Source: three-view drawing plus pictorial views. Frame: mm from the lowest corner of the part. A direction names the side the tool comes from. Give positions to 0.01 mm unless a question says otherwise; leave off trailing zeros. Loops run counter-clockwise (first coordinate to the right, second up) from the corner with the lowest first, then second, coordinate; pieces in that order, holes last. Notation, with made-up numbers: (-25.75, -28) -> (-13.75, -28) arc R26 cw to (-13.75, 5) -> close; hole circle Ø3 at (17.5, 43.5). An arc over 180 degrees is marked (long way). Put each result on its own line as item: value.
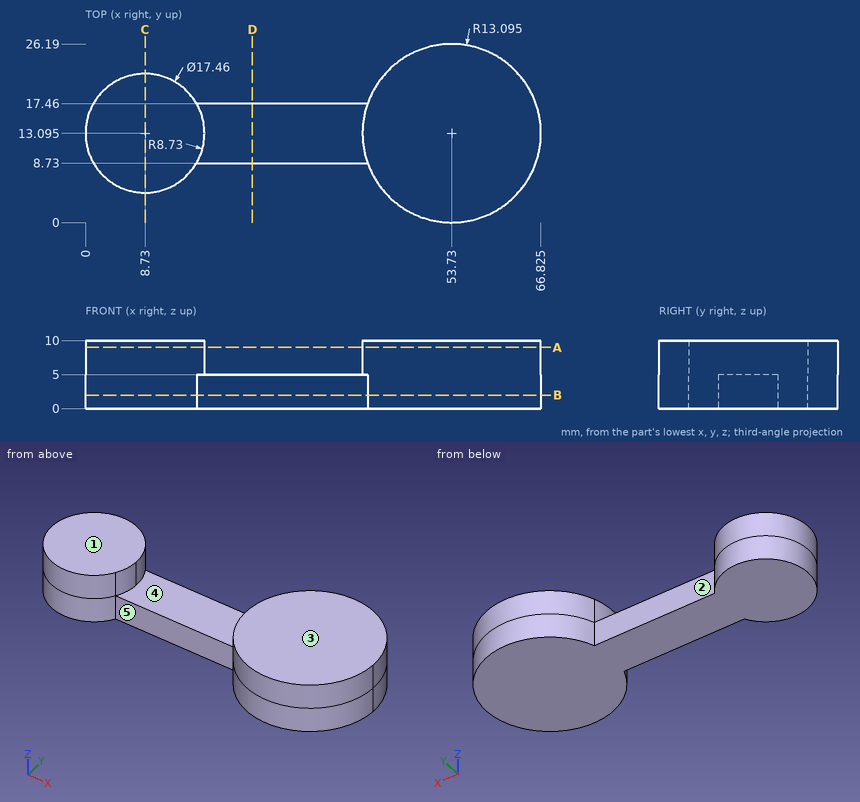
(1) Section D-D on x = 24.5. Return loops of the section in (y, z), then the cut area to 4 significant figures.
Calculated:
outline: (8.73, 0) -> (17.46, 0) -> (17.46, 5) -> (8.73, 5) -> close
area: 43.65 mm²
(2) First-contact query: P1, Ø1, axis at y = 11, z = 4, coming from the -X side; P2, Ø4, axis at x = 27, z = 3, coming from the -Y side; P3, Ø1, axis at x = 48.5, z = 9, coming from the +Y side; P4, Ø2, axis at x = 51.5, y = 5, coming from the -Z side. Flat tips, straight axial feed; report the tip coordinate or a pass-through.
Calculated:
P1: stops at x = 0.15
P2: stops at y = 8.73
P3: stops at y = 25.31
P4: stops at z = 0
(3) Section B-B on z = 2. Return loops of the section in (x, y) (3 decimals), then the cut area to 3 significant figures.
Calculated:
outline: (16.29, 8.73) -> (41.384, 8.73) arc R13.095 ccw (long way) to (41.384, 17.46) -> (16.29, 17.46) arc R8.73 ccw (long way) to start
area: 986 mm²
(4) Section A-A on z = 9. Return loops of the section in (x, y) (3 decimals).
Calculated:
outline: circle Ø17.46 at (8.73, 13.095); circle Ø26.19 at (53.73, 13.095)
(5) Draft query along X for the marked faces 3, 4 and 5. Return one class per face: released by +X, released by -X, zero draft, split by the parting line, or undercut.
Calculated:
face 3: zero draft
face 4: undercut
face 5: undercut
(6) Line query: probe 1 along Z at (x, y) = (31.5, 10.5); probe 2 along X at (y, z) = (12.75, 1); probe 3 along X at (y, z) = (19.25, 8). Output: solid intervals per line, ascending. Write a range as from..to.
Calculated:
probe 1: z = 0..5
probe 2: x = 0.01..66.82
probe 3: x = 2.54..14.92, 42.17..65.29
(7) Reachability of the marked faces 1 and 2 from +Z, -Z, +X, -X, +Y, -Y: full face, straight path, thin tool, end or side. Return the list, or none.
Calculated:
face 1: +Z, +X, -X, +Y, -Y
face 2: +Z, -Z, +Y
(8) Section C-C on x = 8.73. Return loops of the section in (y, z) (3 decimals), then the cut area to 3 significant figures.
Calculated:
outline: (4.365, 0) -> (21.825, 0) -> (21.825, 10) -> (4.365, 10) -> close
area: 175 mm²
